The model under review builds one solid part; all positions refer to its coordinate system, in mm. Coordinates: 2 decimals unless noted, no trailing zeros. Loops run counter-clockwise (first coordinate to the right, second up) from the corner with the lowest first, then second, coordinate; pieces in that order, holes last. Notation, with made-up numbers: (77.25, 83.25) - (92.25, 83.25) arc R23 ccw to (92.25, 112.25) - close; hole circle Ø6 at (49, 5). An arc over 180 degrees is marked (long way). Answer in a Markdown table with one row per item. Add a question column.
(1) Mouldability with a two-part tool opening along X and no side actions: class faces 1 (the flat face through (0, -93, 58.61)), 2 (the cylindrical face through (-0.45, -85.6, 59.39)), 3 (the flat face through (7.24, -91.22, 59.39)) as +X half, -X half, draft (parallel to the pull), parting line (faces both ways), or undercut.
(2) We need section C-C on z = 59.5. Write out the cut boundary in (x, y), plus the area to 3 significant figures.
(3) For line 1 along Y through (x, z) = (0, 59.65); line 2 along Y through (x, z) = (-1.75, 59.6); line 3 along X through (y, z) = (-105.5, 59.7), list the stretches that pass through material, from the lowest coordinate up.
(4) We need section B-B on y = -108. Write out the cut boundary in (x, z), plus the area to 3 significant figures.
(5) We need section A-A on x = -1.25. Write out the cut boundary in (y, z), plus the area to 3 significant figures.
(6) We need section D-D on x = 1.5. Write out the cut boundary in (y, z).
from build123d import *

# Parameters (mm, degrees)
BOSS_EXTRUDE1_DEPTH      = 76.2
BOSS_EXTRUDE1_DEPTH_BACK = 76.2
CUT_EXTRUDE1_DEPTH       = 136.619651209
CUT_EXTRUDE1_DEPTH_BACK  = 136.619651209
FILLET1_R                = 3.81
SHELL1_START             = -44.45
SHELL1_DEPTH             = 88.773
SHELL1_START_2           = -73.025
SHELL1_2_DEPTH           = 130.048
CUT_EXTRUDE2_DEPTH       = 136.355460931
CUT_EXTRUDE2_DEPTH_BACK  = 136.355460931
SKETCH8_W                = 51.042359072
SKETCH8_H                = 158.808122299
CUT_EXTRUDE3_DEPTH       = 112.770943321
CUT_EXTRUDE3_DEPTH_BACK  = 112.770943321
SKETCH9_R                = 2.127


# Read off the part's stored shape, not the designer's step: Shell1
with BuildPart() as part:
    # Sketch1 → Boss-Extrude1 (new, two sides: drawn at the far end of the back side and taken through both)
    with BuildSketch(Plane.XY.offset(-BOSS_EXTRUDE1_DEPTH_BACK)):
        with BuildLine():
            Line((-6.335258536, -105.245804705), (-12.685258536, -3.645804705))
            ThreePointArc((-12.685258536, -3.645804705), (0.014741464, 8.866413132), (12.714741464, -3.645804705))
            Line((12.714741464, -3.645804705), (6.364741464, -105.245804705))
            ThreePointArc((6.364741464, -105.245804705), (0.014741464, -111.465623147), (-6.335258536, -105.245804705))
        make_face()
    extrude(amount=BOSS_EXTRUDE1_DEPTH + BOSS_EXTRUDE1_DEPTH_BACK)

    # Sketch4 → Cut-Extrude1 (cut, two sides: drawn at the far end of the back side and taken through both)
    with BuildSketch(Plane(origin=(0, 0, 0), x_dir=(0, 0, -1), z_dir=(1, 0, 0)).offset(-CUT_EXTRUDE1_DEPTH_BACK)):
        Polygon((-47.498, -73.524605007), (-47.498, -51.299605007), (47.625, -51.299605007), (47.625, -73.524605007), (76.2, -73.524605007), (76.2, 8.866413132), (-76.2, 8.866413132), (-76.2, -28.682279346), (-76.2, -111.465623147), (-60.198, -111.465623147), (-60.198, -73.524605007), align=None)
    extrude(amount=CUT_EXTRUDE1_DEPTH + CUT_EXTRUDE1_DEPTH_BACK, mode=Mode.SUBTRACT)

    # Fillet1
    fillet1_edges = [part.edges().sort_by_distance(p)[0] for p in [
        (8.347316445, -73.524605007, 53.848),
        (9.736378945, -51.299605007, -0.0635),
        (-9.706896017, -51.299605007, -0.0635),
        (-8.317833517, -73.524605007, 53.848),
        (-8.317833517, -73.524605007, -61.9125),
        (8.347316445, -73.524605007, -61.9125),
    ]]
    fillet(fillet1_edges, radius=FILLET1_R)

    # Shell1 outline → Shell1 (cut)
    with BuildSketch(Plane.XY.offset(SHELL1_START)):
        with BuildLine():
            ThreePointArc((-3.161602106, -105.125185529), (0.014741465, -108.290623147), (3.191085035, -105.125185529))
            Line((3.191085035, -105.125185529), (6.314583179, -55.149215219))
            ThreePointArc((6.314583179, -55.149215219), (6.143625088, -54.674822007), (5.680819792, -54.474605007))
            Line((5.680819792, -54.474605007), (-5.651336863, -54.474605007))
            ThreePointArc((-5.651336863, -54.474605007), (-6.114142159, -54.674822006), (-6.285100251, -55.149215219))
            Line((-6.285100251, -55.149215219), (-3.161602106, -105.125185529))
        make_face()
    extrude(amount=SHELL1_DEPTH, mode=Mode.SUBTRACT)

    # Shell1 2 outline → Shell1 2 (cut)
    with BuildSketch(Plane.XY.offset(SHELL1_START_2)):
        with BuildLine():
            Line((-4.896037751, -77.374215219), (-3.161602106, -105.125185529))
            ThreePointArc((-3.161602106, -105.125185529), (0.014741465, -108.290623147), (3.191085035, -105.125185529))
            Line((3.191085035, -105.125185529), (4.925520679, -77.374215219))
            ThreePointArc((4.925520679, -77.374215219), (4.754562588, -76.899822007), (4.291757292, -76.699605007))
            Line((4.291757292, -76.699605007), (-4.262274363, -76.699605007))
            ThreePointArc((-4.262274363, -76.699605007), (-4.725079659, -76.899822006), (-4.896037751, -77.374215219))
        make_face()
    extrude(amount=SHELL1_2_DEPTH, mode=Mode.SUBTRACT)

    # Sketch8 → Cut-Extrude2 (cut, two sides: drawn at the far end of the back side and taken through both)
    with BuildSketch(Plane(origin=(0, 0, 0), x_dir=(1, 0, 0), z_dir=(0, 1, 0)).offset(-CUT_EXTRUDE2_DEPTH_BACK)):
        with Locations((-7.309443233, 20.79356115)):
            Rectangle(SKETCH8_W, SKETCH8_H)
    extrude(amount=CUT_EXTRUDE2_DEPTH + CUT_EXTRUDE2_DEPTH_BACK, mode=Mode.SUBTRACT)

    # Sketch9 → Cut-Extrude3 (cut, two sides: drawn at the far end of the back side and taken through both)
    with BuildSketch(Plane.XY.offset(60.198).offset(-CUT_EXTRUDE3_DEPTH_BACK)):
        with Locations((0.014741464, -106.385623147)):
            Circle(SKETCH9_R)
        with Locations((0.014741464, -83.525623147)):
            Circle(SKETCH9_R)
    extrude(amount=CUT_EXTRUDE3_DEPTH + CUT_EXTRUDE3_DEPTH_BACK, mode=Mode.SUBTRACT)


solid = part.part
Outcome:
| question | item | result |
|---|---|---|
| 1 | face 1 | draft |
| 1 | face 2 | undercut |
| 1 | face 3 | +X half |
| 2 | outline | (-8.06, -77.57) - (-6.34, -105.25) arc R6.35 ccw to (6.36, -105.25) - (8.09, -77.57) arc R3.81 ccw to (4.29, -73.52) - (-4.26, -73.52) arc R3.81 ccw to start; hole circle Ø4.25 at (0.01, -106.39); hole circle Ø4.25 at (0.01, -83.53) |
| 2 | area | 492 mm² |
| 3 | line 1 | -111.47 to -108.51, -104.26 to -85.65, -81.4 to -73.52 |
| 3 | line 2 | -111.22 to -107.57, -105.2 to -84.71, -82.34 to -73.52 |
| 3 | line 3 | -6.32 to -1.92, 1.95 to 6.35 |
| 4 | outline | (-5.64, 58.61) - (-1.37, 58.61) - (-1.37, 60.2) - (-5.64, 60.2) - close; (1.4, 58.61) - (5.67, 58.61) - (5.67, 60.2) - (1.4, 60.2) - close |
| 4 | area | 13.6 mm² |
| 5 | outline | (-111.34, 58.61) - (-108.1, 58.61) - (-108.1, 60.2) - (-111.34, 60.2) - close; (-104.68, 58.61) - (-85.24, 58.61) - (-85.24, 60.2) - (-104.68, 60.2) - close; (-81.82, 58.61) - (-73.52, 58.61) - (-73.52, 60.2) - (-81.82, 60.2) - close |
| 5 | area | 49.2 mm² |
| 6 | outline | (-111.29, 58.61) - (-107.91, 58.61) - (-107.91, 60.2) - (-111.29, 60.2) - close; (-104.86, 58.61) - (-85.05, 58.61) - (-85.05, 60.2) - (-104.86, 60.2) - close; (-82, 58.61) - (-73.52, 58.61) - (-73.52, 60.2) - (-82, 60.2) - close |
